Source: three-view drawing plus pictorial views. Frame: mm from the lowest corner of the part. A direction names the side the tool comes from. Give positions to 0.01 mm unless a question says otherwise; leave off trailing zeros. Loops run counter-clockwise (first coordinate to the right, second up) from the corner with the lowest first, then second, coordinate; pieces in that order, holes last.
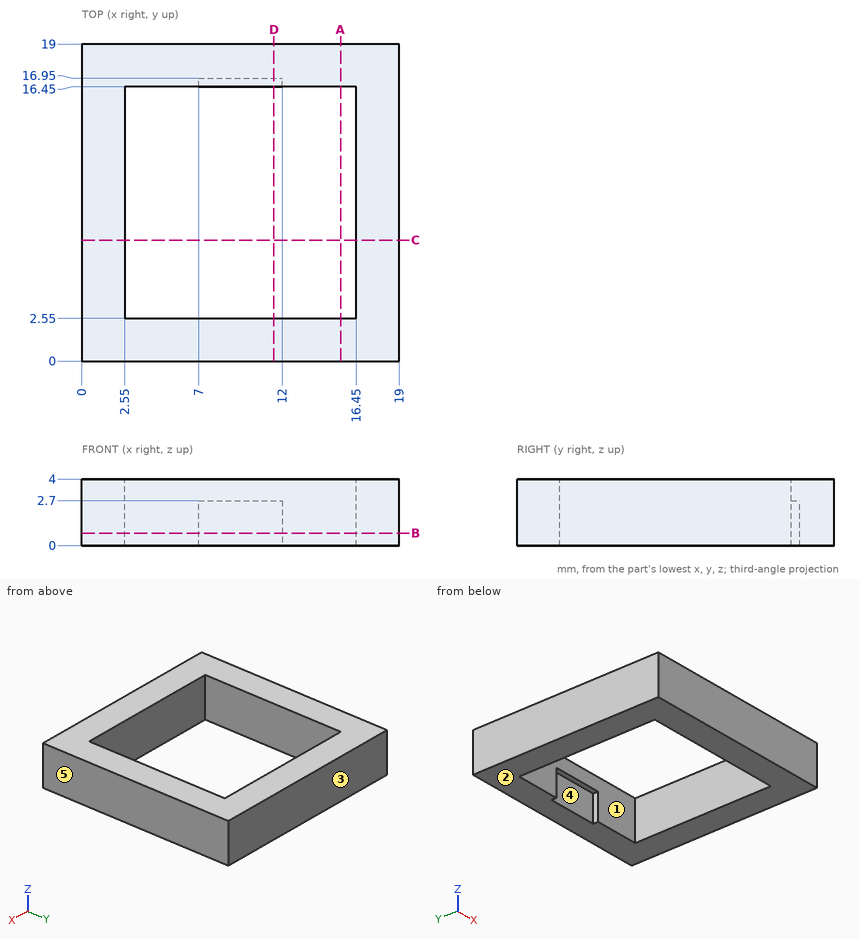
(1) Ray query, probe 1 along X at (y, z) = (15.75, 2.2); probe 2 along Y at (x, z) = (8.25, 1.1). Return the intervals inside material, ascending.
Values follow:
probe 1: x = 0 to 2.55, 16.45 to 19
probe 2: y = 0 to 2.55, 16.95 to 19
(2) Cut plane B-B (z = 0.75). Return the cut outline in (x, y).
Values follow:
outline: (0, 0) - (19, 0) - (19, 19) - (0, 19) - close; hole (2.55, 2.55) - (16.45, 2.55) - (16.45, 16.45) - (12, 16.45) - (12, 16.95) - (7, 16.95) - (7, 16.45) - (2.55, 16.45) - close
(3) Cut plane A-A (x = 15.5). Return the cut outline in (y, z), and give its area (3 significant figures).
Values follow:
outline: (0, 0) - (2.55, 0) - (2.55, 4) - (0, 4) - close; (16.45, 0) - (19, 0) - (19, 4) - (16.45, 4) - close
area: 20.4 mm2
(4) Cut plane D-D (x = 11.5). Return the cut outline in (y, z).
Values follow:
outline: (0, 0) - (2.55, 0) - (2.55, 4) - (0, 4) - close; (16.45, 2.7) - (16.95, 2.7) - (16.95, 0) - (19, 0) - (19, 4) - (16.45, 4) - close
(5) Reachability of the marked faces 1 and 2 from +Z, -Z, +X, -X, +Y, -Y: full face, straight path, thin tool, end or side. Return the list, or none.
Values follow:
face 1: +Z, -Z
face 2: -Z, +X, -X, +Y, -Y
(6) Mould query, pull axis X, two halves, no side actions, for the marked faces 3, 4 and 5. Classes: +X half, -X half, draft (parallel to the pull), parting line (faces both ways), or undercut.
Values follow:
face 3: draft
face 4: undercut
face 5: +X half
